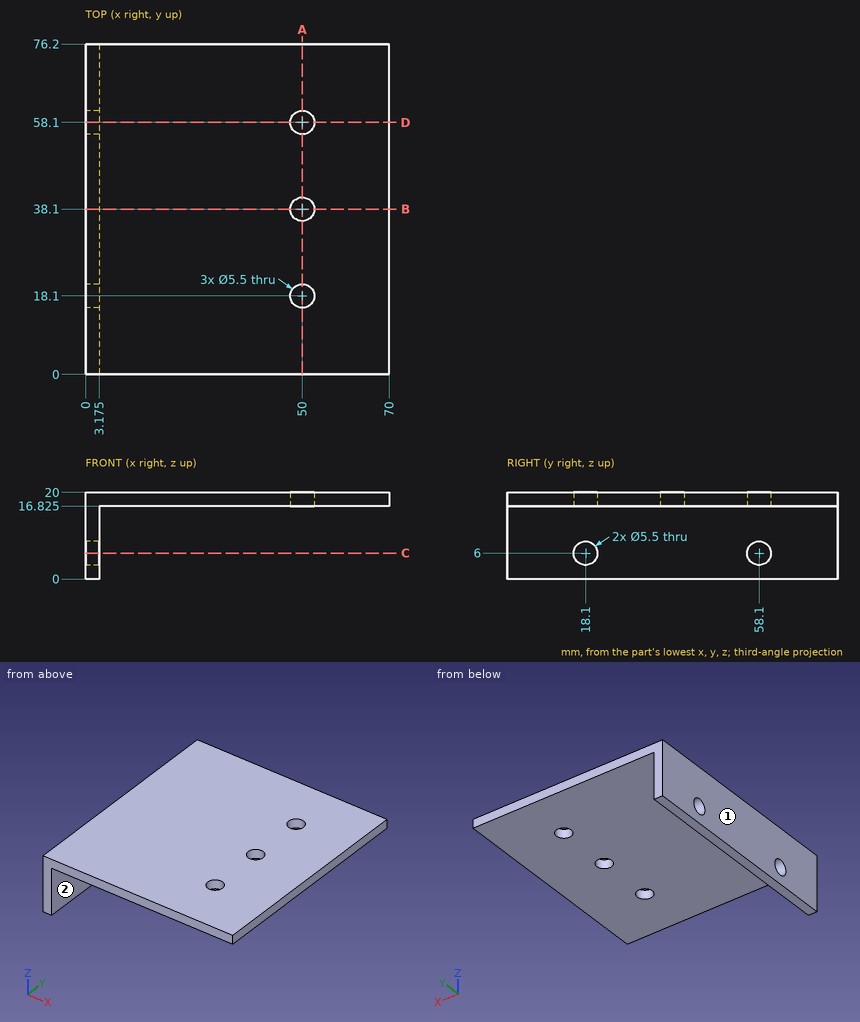
Study the drawing (mm; zero at the part's minimum x, y, z) and answer. A direction names the side the tool comes from. Coordinates: 2 decimals unless noted, no trailing zeros. Loops run counter-clockwise (first coordinate to the right, second up) from the corner with the lowest first, then second, coordinate; pieces in that order, holes last. Notation, with made-up numbers: (31, -13) -> (87, -13) arc R17 ccw to (87, 12) -> close; hole circle Ø7 at (-22, 19). An arc over 180 degrees is marked (long way). Answer in a Markdown table with one row per item. Add a question column.
1. Flat-ended cylindrical pins translate along their axes: P1, Ø4, axis at x = 10.5, z = 13.5, coming from the +Y side; P2, Ø3, axis at y = 31, z = 8.5, coming from the +X side (3 decimals); P3, Ø3, axis at x = 25.5, y = 25, coming from the -Z side (3 decimals). Find the tip coordinate at first contact, or state that the pin passes through.
2. For the marked faces 1 and 2, determine the directions among +Z, -Z, +X, -X, +Y, -Y from which every point of the face is accessible in a straight line to the end or side of a thin tool.
3. The part is cut by section B-B, the plane y = 38.1. Write down the section's boundary in (x, z) (3 decimals).
4. Consider line 1 (Y direction, x = 50, z = 18.85); line 2 (Y direction, x = 2.05, z = 6); line 3 (Z direction, x = 57, y = 70.5) (3 decimals). Determine where each line is inside the solid, lowest interval first. Write a range as [from, to].
5. The part is cut by section C-C, the plane z = 6. Write down the section's boundary in (x, y) (3 decimals).
6. The part is cut by section A-A, the plane x = 50. Write down the section's boundary in (y, z) (3 decimals).
7. The part is cut by section D-D, the plane y = 58.1. Write down the section's boundary in (x, z) (3 decimals), then the cut area to 3 significant figures.
Answer below:
| question | item | result |
|---|---|---|
| 1 | P1 | through |
| 1 | P2 | x = 3.175 |
| 1 | P3 | z = 16.825 |
| 2 | face 1 | +Z, -Z, -X, +Y, -Y |
| 2 | face 2 | -Z, +X, +Y, -Y |
| 3 | outline | (0, 0) -> (3.175, 0) -> (3.175, 16.825) -> (47.25, 16.825) -> (47.25, 20) -> (0, 20) -> close; (52.75, 16.825) -> (70, 16.825) -> (70, 20) -> (52.75, 20) -> close |
| 4 | line 1 | [0, 15.35], [20.85, 35.35], [40.85, 55.35], [60.85, 76.2] |
| 4 | line 2 | [0, 15.35], [20.85, 55.35], [60.85, 76.2] |
| 4 | line 3 | [16.825, 20] |
| 5 | outline | (0, 0) -> (3.175, 0) -> (3.175, 15.35) -> (0, 15.35) -> close; (0, 20.85) -> (3.175, 20.85) -> (3.175, 55.35) -> (0, 55.35) -> close; (0, 60.85) -> (3.175, 60.85) -> (3.175, 76.2) -> (0, 76.2) -> close |
| 6 | outline | (0, 16.825) -> (15.35, 16.825) -> (15.35, 20) -> (0, 20) -> close; (20.85, 16.825) -> (35.35, 16.825) -> (35.35, 20) -> (20.85, 20) -> close; (40.85, 16.825) -> (55.35, 16.825) -> (55.35, 20) -> (40.85, 20) -> close; (60.85, 16.825) -> (76.2, 16.825) -> (76.2, 20) -> (60.85, 20) -> close |
| 7 | outline | (0, 0) -> (3.175, 0) -> (3.175, 3.25) -> (0, 3.25) -> close; (0, 8.75) -> (3.175, 8.75) -> (3.175, 16.825) -> (47.25, 16.825) -> (47.25, 20) -> (0, 20) -> close; (52.75, 16.825) -> (70, 16.825) -> (70, 20) -> (52.75, 20) -> close |
| 7 | area | 241 mm2 |
